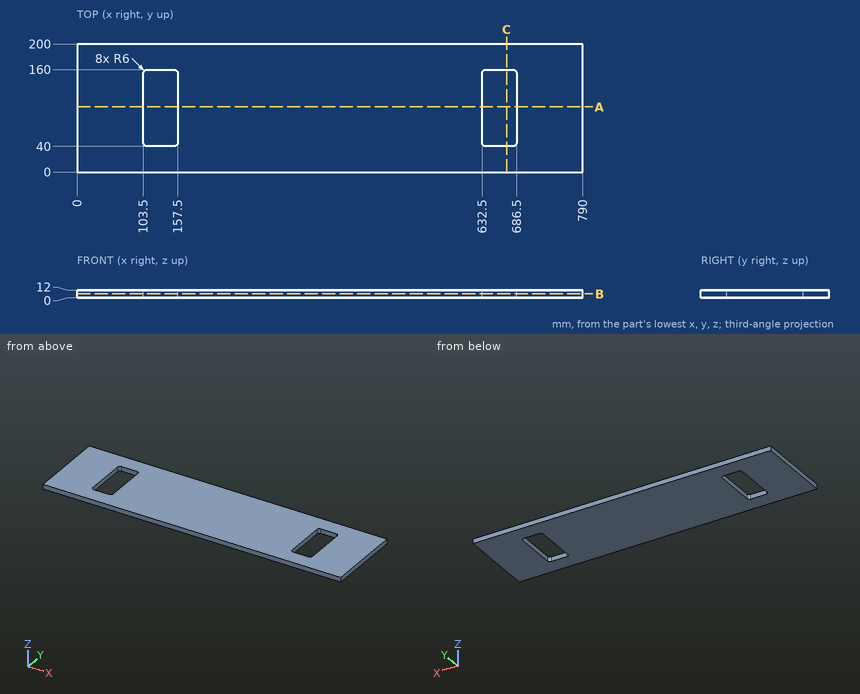
Study the drawing (mm; zero at the part's minimum x, y, z) and answer. Give positions to 0.01 mm unless a question says otherwise; leave off trailing zeros. Write each loop counter-clockwise with the first axis right and the second up, starting at its lowest first coordinate (ties: lowest second). Pieces come first, ordered by that corner, then holes. Notation, with made-up numbers: (-38.75, 75) -> (-20.75, 75) arc R6 ccw to (-20.75, 80) -> close; hole circle Ø6 at (77, -35.5). An arc over 180 degrees is marked (long way). Write item = value, one per line.
Q1. A flat-ended cylindrical pin translates along its axis: pin 1 Ø8 at (x, y) = (121, 43) entering from +Z. Find the tip coordinate at first contact, or state that the pin passes through.
Computed values:
pin_1 = 12
Q2. Section A-A on y = 102 is taken. Determine the outline of the cut face in (x, z), and give its area (3 significant figures).
Computed values:
outline = (0, 0) -> (103.5, 0) -> (103.5, 12) -> (0, 12) -> close; (157.5, 0) -> (632.5, 0) -> (632.5, 12) -> (157.5, 12) -> close; (686.5, 0) -> (790, 0) -> (790, 12) -> (686.5, 12) -> close
area = 8,180 mm^2
Q3. Section B-B on z = 6 is taken. Determine the outline of the cut face in (x, y), and give its area (3 significant figures).
Computed values:
outline = (0, 0) -> (790, 0) -> (790, 200) -> (0, 200) -> close; hole (103.5, 46) arc R6 ccw to (109.5, 40) -> (151.5, 40) arc R6 ccw to (157.5, 46) -> (157.5, 154) arc R6 ccw to (151.5, 160) -> (109.5, 160) arc R6 ccw to (103.5, 154) -> close; hole (632.5, 46) arc R6 ccw to (638.5, 40) -> (680.5, 40) arc R6 ccw to (686.5, 46) -> (686.5, 154) arc R6 ccw to (680.5, 160) -> (638.5, 160) arc R6 ccw to (632.5, 154) -> close
area = 145,000 mm^2
Q4. Section C-C on x = 671 is taken. Determine the outline of the cut face in (y, z), and give its area (3 significant figures).
Computed values:
outline = (0, 0) -> (40, 0) -> (40, 12) -> (0, 12) -> close; (160, 0) -> (200, 0) -> (200, 12) -> (160, 12) -> close
area = 960 mm^2
Q5. Consider line 1 along X through (y, z) = (51, 1); line 2 along Y through (x, z) = (671.5, 10.25); line 3 along Y through (x, z) = (635.5, 9.25). Determine where each line is inside the solid, lowest interval first.
Computed values:
line_1 = 0 to 103.5, 157.5 to 632.5, 686.5 to 790
line_2 = 0 to 40, 160 to 200
line_3 = 0 to 40.8, 159.2 to 200
